Answer from the drawing. Dimensions are ordinates in mm from the lowest x, y and z of the part. Round coordinates to 2 decimals unless told otherwise and drop trailing zeros. Loops run counter-clockwise (first coordinate to the right, second up) from the corner with the lowest first, then second, coordinate; pieces in that order, holes last.
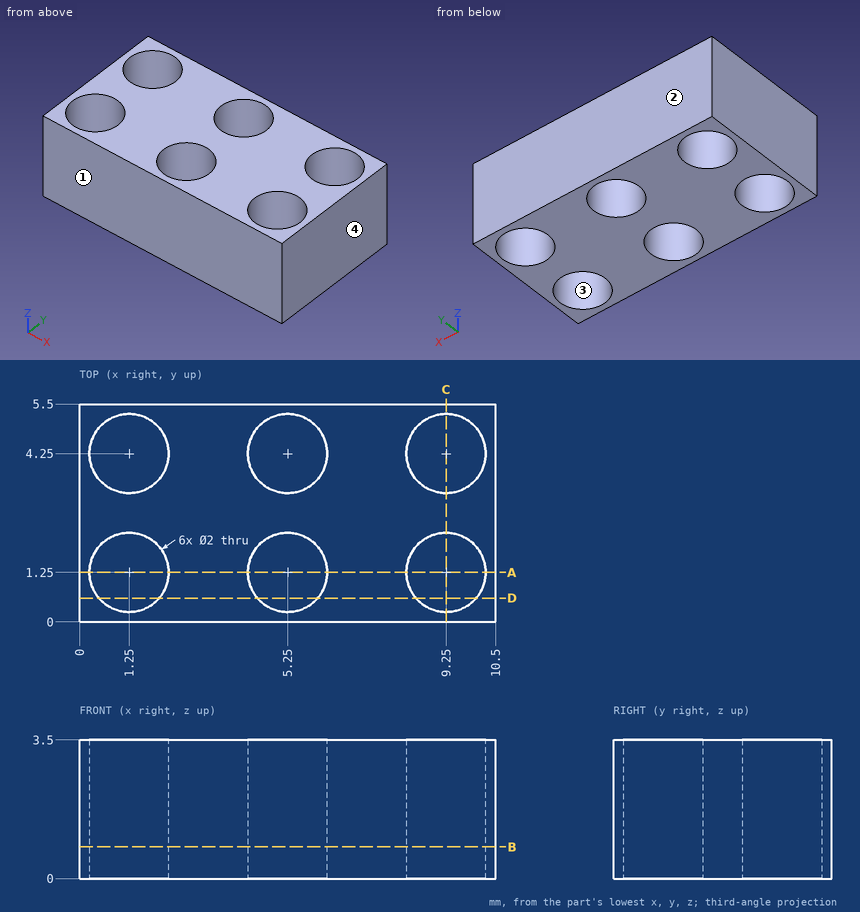
1. Find section A-A (y = 1.25). Write down the section's boundary in (x, z).
Answer key:
outline: (0, 0) - (0.25, 0) - (0.25, 3.5) - (0, 3.5) - close; (2.25, 0) - (4.25, 0) - (4.25, 3.5) - (2.25, 3.5) - close; (6.25, 0) - (8.25, 0) - (8.25, 3.5) - (6.25, 3.5) - close; (10.25, 0) - (10.5, 0) - (10.5, 3.5) - (10.25, 3.5) - close
2. Find section C-C (x = 9.25). Write down the section's boundary in (y, z).
Answer key:
outline: (0, 0) - (0.25, 0) - (0.25, 3.5) - (0, 3.5) - close; (2.25, 0) - (3.25, 0) - (3.25, 3.5) - (2.25, 3.5) - close; (5.25, 0) - (5.5, 0) - (5.5, 3.5) - (5.25, 3.5) - close
3. Determine the mould class of the marked faces 1, 2, 3 and 4 for opening direction Y: +Y half, -Y half, draft (parallel to the pull), parting line (faces both ways), or undercut.
Answer key:
face 1: -Y half
face 2: +Y half
face 3: undercut
face 4: draft
4. Find section B-B (z = 0.8). Write down the section's boundary in (x, y).
Answer key:
outline: (0, 0) - (10.5, 0) - (10.5, 5.5) - (0, 5.5) - close; hole circle Ø2 at (1.25, 1.25); hole circle Ø2 at (1.25, 4.25); hole circle Ø2 at (5.25, 1.25); hole circle Ø2 at (5.25, 4.25); hole circle Ø2 at (9.25, 1.25); hole circle Ø2 at (9.25, 4.25)
5. Consider probe 1 along Y at (x, z) = (5.25, 1.95); probe 2 along X at (y, z) = (4.25, 2.65); probe 3 along Y at (x, z) = (8.5, 3). Determine where each line is inside the solid, lowest interval first.
Answer key:
probe 1: y = 0 to 0.25, 2.25 to 3.25, 5.25 to 5.5
probe 2: x = 0 to 0.25, 2.25 to 4.25, 6.25 to 8.25, 10.25 to 10.5
probe 3: y = 0 to 0.59, 1.91 to 3.59, 4.91 to 5.5
6. Find section D-D (y = 0.6). Write down the section's boundary in (x, z).
Answer key:
outline: (0, 0) - (0.49, 0) - (0.49, 3.5) - (0, 3.5) - close; (2.01, 0) - (4.49, 0) - (4.49, 3.5) - (2.01, 3.5) - close; (6.01, 0) - (8.49, 0) - (8.49, 3.5) - (6.01, 3.5) - close; (10.01, 0) - (10.5, 0) - (10.5, 3.5) - (10.01, 3.5) - close
